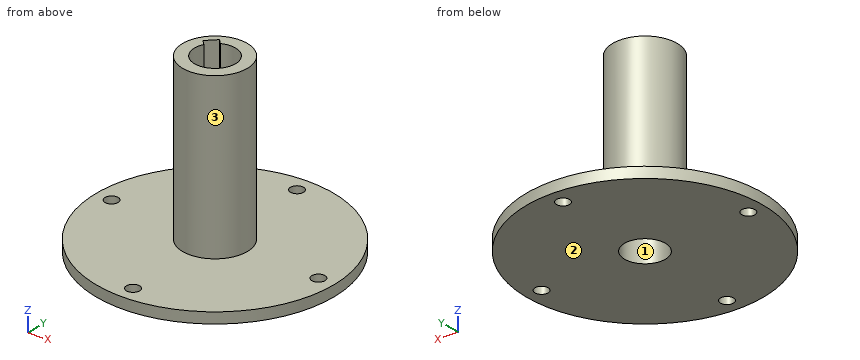
Autodesk Inventor part; units mm, degrees
ref_plane "YZ Plane" through (0, 0, 0) normal (1, 0, 0) x (0, 1, 0)
ref_plane "XZ Plane" through (0, 0, 0) normal (0, 1, 0) x (-1, 0, 0)
ref_plane "XY Plane" through (0, 0, 0) normal (0, 0, 1) x (1, 0, 0)
sketch "Sketch1" plane through (0, 0, 0) normal (0, 0, 1) x (1, 0, 0)
  circle A0 centre (0, 0) radius 47.5 construction
  circle A1 centre (0, 47.5) radius 3.05
  circle A2 centre (-47.5, 0) radius 3.05
  circle A3 centre (0, -47.5) radius 3.05
  circle A4 centre (47.5, 0) radius 3.05
  circle A5 centre (0, 0) radius 15 construction
  circle A6 centre (0, 0) radius 55
  circle A7 centre (0, 0) radius 9.5
  dimension "d0" = 95
  dimension "d1" = 6.1
  dimension "d4" = 360
  dimension "d6" = 30
  dimension "d7" = 110
  dimension "d8" = 19
extrude "Extrusion1" add sketch "Sketch1" along normal blind 5
sketch "Sketch2" plane through (0, 0, 5) normal (0, 0, 1) x (1, 0, 0)
  circle A0 centre (0, 0) radius 15
  circle A1 centre (0, 0) radius 9.5
  dimension "d11" = 30
extrude "Extrusion2" add sketch "Sketch2" along normal blind 75
sketch "Sketch3" plane through (0, 0, 80) normal (0, 0, 1) x (1, 0, 0)
  circle A0 centre (0, 0) radius 15
  circle A1 centre (0, 0) radius 9.5
  line L0 (6.7175, -6.7175) -> (-8.4853, 8.4853)
  line L1 (-8.4853, 8.4853) -> (-10.6066, 6.364)
  line L2 (-10.6066, 6.364) -> (-8.4951, 4.2525)
  line L3 (-8.4853, 8.4853) -> (-6.364, 10.6066)
  line L4 (-6.364, 10.6066) -> (-4.2525, 8.4951)
  dimension "d14" = 21.5
  dimension "d15" = 3
  dimension "d16" = 3
extrude "Extrusion3" cut sketch "Sketch3" against normal blind 40 contours A1 L0 L3 L4 | A1 L2 L1 L0
properties part number "wheelFlangeTopMotor"
Read the model definition and answer for the solid it produces. Units are mm, in the model's axes. Face numbers are marked on the shaded views. Give positions to 0.01 mm unless a question says otherwise; leave off trailing zeros. Write each loop counter-clockwise with the first axis right and the second up, starting at its lowest first coordinate (ties: lowest second). Pieces come first, ordered by that corner, then holes. Notation, with made-up numbers: (75.25, 37.5) -> (101.25, 37.5) arc R21 cw to (101.25, 74.5) -> close; hole circle Ø3 at (-34, -6.5). An arc over 180 degrees is marked (long way). Answer as a JSON object with one key per item and string values.
1) Straight lines are drawn through the part: probe 1 along Y at (x, z) = (0, 1.5); probe 2 along Y at (x, z) = (0, 28); probe 3 along Z at (x, y) = (-38, 6.5). For each, find the intervals that lie inside material, in ascending order. Write a range as from..to.
Findings below:
{"probe 1": "y = -55..-50.55, -44.45..-9.5, 9.5..44.45, 50.55..55", "probe 2": "y = -15..-9.5, 9.5..15", "probe 3": "z = 0..5"}
2) Flat-ended cylindrical pins translate along their axes: pin 1 Ø3.5 at (x, y) = (0, -47.5) entering from -Z; pin 2 Ø12 at (x, z) = (-13.5, 60) entering from +Y; pin 3 Ø4 at (x, z) = (3.5, 34) entering from +Y; pin 4 Ø1.9 at (x, y) = (-6.5, 8) entering from +Z. Find the tip coordinate at first contact, or state that the pin passes through.
Findings below:
{"pin 1": "passes through", "pin 2": "stops at y = 12.99", "pin 3": "stops at y = 14.92", "pin 4": "stops at z = 40"}
3) For a pull along Y with two mould halves and no side action, classify the marked faces 1, 2 and 3 as pulls with the +Y half, pulls with the -Y half, needs draft (parallel to the pull), parting line crosses it, or undercut.
Findings below:
{"face 1": "undercut", "face 2": "needs draft", "face 3": "parting line crosses it"}
4) Section C-C on y = 47.5 is taken. Write down the section's boundary in (x, z).
Findings below:
{"outline": "(-27.73, 0) -> (-3.05, 0) -> (-3.05, 5) -> (-27.73, 5) -> close; (3.05, 0) -> (27.73, 0) -> (27.73, 5) -> (3.05, 5) -> close"}
5) Section A-A on y = 0 is taken. Write down the section's boundary in (x, z).
Findings below:
{"outline": "(-55, 0) -> (-50.55, 0) -> (-50.55, 5) -> (-55, 5) -> close; (-44.45, 0) -> (-9.5, 0) -> (-9.5, 80) -> (-15, 80) -> (-15, 5) -> (-44.45, 5) -> close; (9.5, 0) -> (44.45, 0) -> (44.45, 5) -> (15, 5) -> (15, 80) -> (9.5, 80) -> close; (50.55, 0) -> (55, 0) -> (55, 5) -> (50.55, 5) -> close"}
